from build123d import *

# Parameters (mm, degrees)
CYLINDER005_R          = 5
CYLINDER005_DEPTH      = 3
CYLINDER003_R          = 2
CYLINDER003_DEPTH      = 4
CYLINDER002_R          = 2
CYLINDER002_DEPTH      = 2
CUT001_PLACEMENT_ANGLE = 180
CYLINDER001_R          = 2
CYLINDER001_DEPTH      = 4
CYLINDER_R             = 2
CYLINDER_DEPTH         = 2
CYLINDER004_R          = 6
CYLINDER004_DEPTH      = 2


with BuildPart() as cylinder005:
    # Cylinder005 → Cylinder005 (new body)
    with BuildSketch(Plane(origin=(5, 5, 0), x_dir=(1, 0, 0), z_dir=(0, 0, 1))):
        Circle(CYLINDER005_R)
    extrude(amount=CYLINDER005_DEPTH)


with BuildPart() as cylinder003:
    # Cylinder003 → Cylinder003 (new body)
    with BuildSketch(Plane(origin=(0, 1.5, 0), x_dir=(1, 0, 0), z_dir=(0, 0, 1))):
        Circle(CYLINDER003_R)
    extrude(amount=CYLINDER003_DEPTH)


with BuildPart() as cut001:
    # Cylinder002 → Cylinder002 (new body)
    with BuildSketch(Plane.XY):
        Circle(CYLINDER002_R)
    extrude(amount=CYLINDER002_DEPTH)

    # Cut001: cut Cylinder003
    add(cylinder003.part, mode=Mode.SUBTRACT)


with BuildPart() as cut001_1:
    # Cut001 placement: moved
    add(cut001.part.moved(Location((0, 10, 0))).rotate(Axis((0, 10, 0), (0, 0, 1)), CUT001_PLACEMENT_ANGLE))


with BuildPart() as cylinder001:
    # Cylinder001 → Cylinder001 (new body)
    with BuildSketch(Plane(origin=(0, 1.5, 0), x_dir=(1, 0, 0), z_dir=(0, 0, 1))):
        Circle(CYLINDER001_R)
    extrude(amount=CYLINDER001_DEPTH)


with BuildPart() as cut:
    # Cylinder → Cylinder (new body)
    with BuildSketch(Plane.XY):
        Circle(CYLINDER_R)
    extrude(amount=CYLINDER_DEPTH)

    # Cut: cut Cylinder001
    add(cylinder001.part, mode=Mode.SUBTRACT)


with BuildPart() as cut002:
    # Cylinder004 → Cylinder004 (new body)
    with BuildSketch(Plane(origin=(5, 5, 0), x_dir=(1, 0, 0), z_dir=(0, 0, 1))):
        Circle(CYLINDER004_R)
    extrude(amount=CYLINDER004_DEPTH)

    # Fusion: union Cut001, Cut
    add(cut001_1.part)
    add(cut.part)

    # Cut002: cut Cylinder005
    add(cylinder005.part, mode=Mode.SUBTRACT)


solid = cut002.part
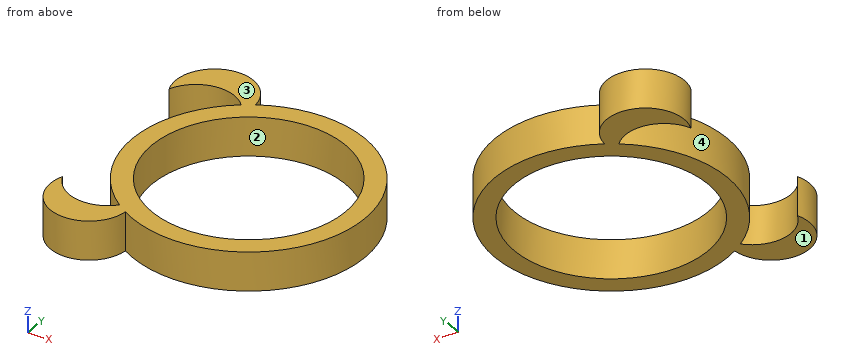
Input: part model. Units: mm. Frame: model coordinates. Face numbers are marked on the shaded views. A direction names the side the tool comes from. Give positions to 0.01 mm unless a question says otherwise; leave off trailing zeros. Order: outer loops, then holes, each group sorted by start corner. A loop starts at its lowest first (then second) coordinate and runs counter-clockwise, first axis right, second up.
Q1. Ray query, probe 1 along Y at (x, z) = (5, 0.65); probe 2 along X at (y, z) = (7, 1.25). Return the intervals inside material, ascending.
Checked values:
probe 1: y = -1 to 0, 10 to 11
probe 2: x = -0.66 to 0.42, 9.58 to 10.66
Q2. Set-up query: the marked faces 3 and 4. Return all of +Z, -Z, +X, -X, +Y, -Y with unobstructed straight access to the full face (end or side cutting, diameter ignored); none if empty.
Checked values:
face 3: +Z, +X, -X, +Y, -Y
face 4: +Z, -Z
Q3. Draft query along X for the marked faces 1 and 2. Return one class per face: +X half, -X half, draft (parallel to the pull), parting line (faces both ways), or undercut.
Checked values:
face 1: draft
face 2: undercut
Q4. Section C-C on x = -0.25. Output: boundary loops of the cut face in (y, z), and give its area (3 significant figures).
Checked values:
outline: (-1.98, 0) - (-0.48, 0) - (-0.48, 2) - (-1.98, 2) - close; (2.1, 0) - (7.9, 0) - (7.9, 2) - (2.1, 2) - close; (10.48, 0) - (11.98, 0) - (11.98, 2) - (10.48, 2) - close
area: 17.6 mm2
Q5. Section A-A on x = 5. Output: boundary loops of the cut face in (y, z).
Checked values:
outline: (-1, 0) - (0, 0) - (0, 2) - (-1, 2) - close; (10, 0) - (11, 0) - (11, 2) - (10, 2) - close
Q6. Contact query for flat-ended pins moving along their axis: pin 1 Ø1 at (x, z) = (6, 1.5) entering from +Y; pin 2 Ø4 at (x, y) = (4, 7.5) entering from -Z. Output: stop coordinate, or through.
Checked values:
pin 1: stops at y = 10.98
pin 2: passes through
Q7. Section D-D on z = 0.6. Output: boundary loops of the cut face in (x, y).
Checked values:
outline: (-1.85, 0.75) arc R2 ccw (long way) to (1.99, -0.19) arc R6 ccw (long way) to (1.99, 10.19) arc R2 ccw (long way) to (-1.85, 9.25) arc R2 cw to (1.47, 9.85) arc R6 ccw to (1.47, 0.15) arc R2 cw to start; hole circle Ø10 at (5, 5)
